```python
from build123d import *

# Parameters (mm, degrees)
SKETCH_1_W          = 20
SKETCH_1_H          = 24
SKETCH_1_W_2        = 12
SKETCH_1_H_2        = 16
EXTRUDE_1_DEPTH     = 4
SKETCH_2_W          = 20
SKETCH_2_H          = 3
EXTRUDE_2_DEPTH     = 8
EXTRUDE_3_DEPTH     = 4
SKETCH_4_R          = 2.1
CUT_EXTRUDE_1_DEPTH = 26
FILLET_1_R          = 2
FILLET_4_R          = 2


with BuildPart() as part:
    # 草图1 → 凸台-拉伸1 (new body)
    with BuildSketch(Plane.XY):
        with Locations((6, 8)):
            Rectangle(SKETCH_1_W, SKETCH_1_H)
        with Locations((6, 8)):
            Rectangle(SKETCH_1_W_2, SKETCH_1_H_2, mode=Mode.SUBTRACT)
    extrude(amount=EXTRUDE_1_DEPTH)

    # 草图2 → 凸台-拉伸2 (add)
    with BuildSketch(Plane.ZY.offset(4)):
        with Locations((2, 3.5)):
            Rectangle(SKETCH_2_W, SKETCH_2_H)
    extrude(amount=EXTRUDE_2_DEPTH)

    # 草图3 → 凸台-拉伸3 (add)
    with BuildSketch(Plane.XY.offset(4)):
        Polygon((-12, 5), (-4, 20), (-4, 5), align=None)
    extrude(amount=-EXTRUDE_3_DEPTH)

    # 草图4 → 切除-拉伸1 (cut, through all)
    with BuildSketch(Plane(origin=(0, 5, 0), x_dir=(1, 0, 0), z_dir=(0, 1, 0))):
        with Locations(Location((-8, 4, 0), (0, 0, 270))):
            Circle(SKETCH_4_R)
        with Locations(Location((-8, -8, 0), (0, 0, 270))):
            Circle(SKETCH_4_R)
    extrude(amount=-CUT_EXTRUDE_1_DEPTH, mode=Mode.SUBTRACT)

    # 圆角1
    fillet_1_edges = [part.edges().sort_by_distance(p)[0] for p in [
        (0, 16, 2),
        (0, 0, 2),
        (12, 0, 2),
        (12, 16, 2),
    ]]
    fillet(fillet_1_edges, radius=FILLET_1_R)

    # 圆角4
    fillet_4_edges = [part.edges().sort_by_distance(p)[0] for p in [
        (-4, 3.5, 0),
        (-4, 3.5, 4),
    ]]
    fillet(fillet_4_edges, radius=FILLET_4_R)


solid = part.part
```
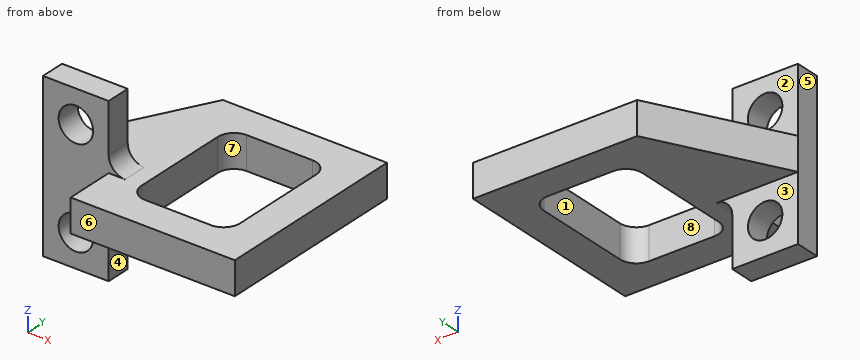
Input: part model. Units: mm. Frame: model coordinates. Face numbers are marked on the shaded views. A direction names the side the tool comes from. Round coordinates to 2 decimals unless told otherwise and drop trailing zeros. Loops run counter-clockwise (first coordinate to the right, second up) from the corner with the lowest first, then second, coordinate; pieces in that order, holes last. Notation, with made-up numbers: (34.5, 22.25) - (76.5, 22.25) arc R27 ccw to (76.5, 45.25) - close; hole circle Ø4 at (47.5, 58.5). An arc over 180 degrees is marked (long way). One line per item, written item: value. Start each with the question number.
(1) Section B-B, the plane x = 8. Return loops of the section in (y, z).
(2) Contact query for flat-ended pins moving along their axis: P1, Ø6, axis at x = -5.5, y = 17.5, coming from the -Z side; P2, Ø12, axis at x = -2, y = 2.5, coming from the -Z side; P3, Ø8, axis at y = 11.5, z = 0.5, coming from the -X side; P4, Ø6.5, axis at x = -8, z = -4, coming from the +Y side. Output: stop coordinate, or through.
(3) Section A-A, the plane y = 13.25. Return loops of the section in (x, z).
(4) Section D-D, the plane x = -7.25. Return loops of the section in (y, z), plus the area to 3 significant figures.
(5) Draft query along Y for the marked faces 5, 6, 7 and 8. Return one class per face: +Y half, -Y half, draft (parallel to the pull), parting line (faces both ways), or undercut.
(6) Ray query, line 1 (X direction, y = 2.9, z = 8); line 2 (Z direction, x = -4.75, y = 14.5); line 3 (Y direction, x = -5.5, z = 6.75). Return the intervals inside material, ascending. Write a range as [from, to].
(7) Section C-C, the plane z = 2.75. Return loops of the section in (x, y), plus the area to 3 significant figures.
(8) Access query for the marked faces 1, 2, 3 and 4. Directions: +Z, -Z, +X, -X, +Y, -Y. A direction counts if a zero-diameter tool reaches every point of the face in a straight line with its end or side. Return the directions, or none.
Results below:
1. outline: (-4, 0) - (0, 0) - (0, 4) - (-4, 4) - close; (16, 0) - (20, 0) - (20, 4) - (16, 4) - close
2. P1: z = 0
2. P2: z = -8
2. P3: x = -10.67
2. P4: y = 5
3. outline: (-7.6, 0) - (0, 0) - (0, 4) - (-7.6, 4) - close; (12, 0) - (16, 0) - (16, 4) - (12, 4) - close
4. outline: (2, -8) - (5, -8) - (5, -5.96) - (2, -5.96) - close; (2, -2.04) - (5, -2.04) - (5, 0) - (13.91, 0) - (13.91, 4) - (5, 4) - (5, 6.04) - (2, 6.04) - close; (2, 9.96) - (5, 9.96) - (5, 12) - (2, 12) - close
4. area: 72.1 mm^2
5. face 5: draft
5. face 6: -Y half
5. face 7: undercut
5. face 8: undercut
6. line 1: [-12, -10.1], [-5.9, -4]
6. line 2: [0, 4]
6. line 3: [2, 5]
7. outline: (-12, 2) - (-4, 2) - (-4, -4) - (16, -4) - (16, 20) - (-4, 20) - (-12, 5) - close; hole (0, 2) arc R2 ccw to (2, 0) - (10, 0) arc R2 ccw to (12, 2) - (12, 14) arc R2 ccw to (10, 16) - (2, 16) arc R2 ccw to (0, 14) - close
7. area: 375 mm^2
8. face 1: +Z, -Z
8. face 2: +Z, +X, -X, +Y
8. face 3: -Z, +X, -X, +Y
8. face 4: -Z, +X, +Y, -Y
